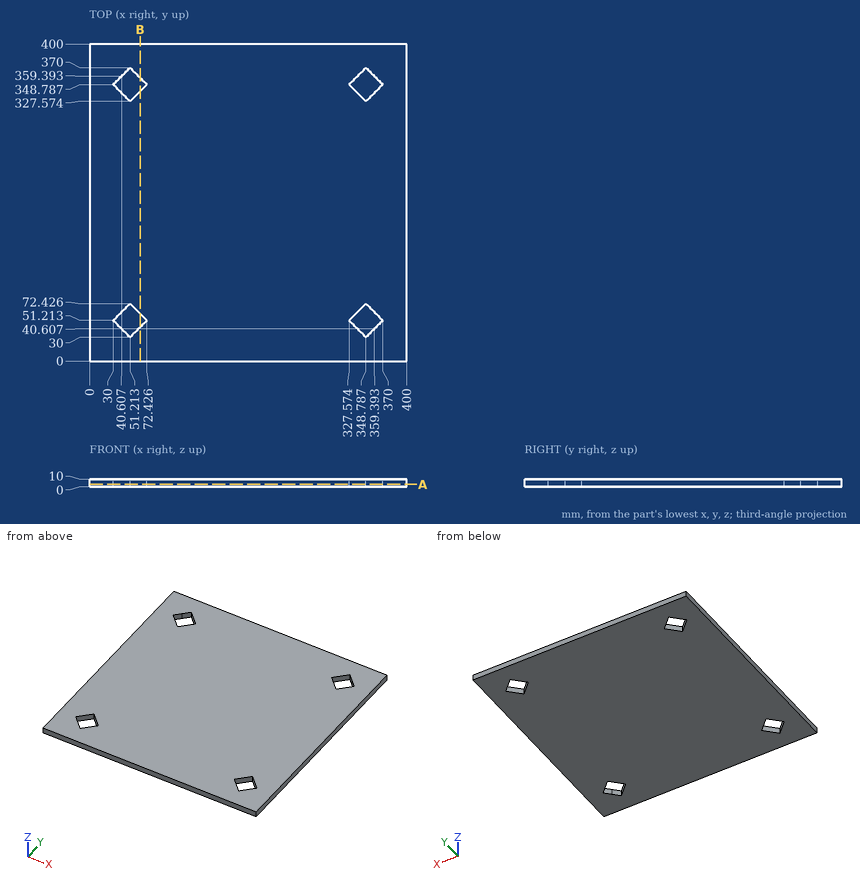
Input: dimensioned drawing with shaded views. Units: mm. Origin: part minimum x, y, z. Give positions to 0.01 mm unless a question says otherwise; leave off trailing zeros. Write each loop counter-clockwise with the first axis right and the second up, starting at its lowest first coordinate (ties: lowest second). Pieces come first, ordered by that corner, then holes. Notation, with made-up numbers: M -8,67 L 21,67 A13 ccw 21,72 Z; hole C 87,21 d7. An arc over 180 degrees is marked long. Return JSON: item names as keys, results as strings. Group by question number.
1) Cut plane B-B, the plane x = 64. Output: boundary loops of the cut face in (y, z).
2) Cut plane A-A, the plane z = 3.25. Output: boundary loops of the cut face in (x, y), plus the area to 3 significant figures.
3) Material intervals for line 1 along Y through (x, z) = (33, 6) (1 decimal); line 2 along Y through (x, z) = (37, 6.5) (1 decimal); line 3 along X through (y, z) = (350.5, 1) (1 decimal), sorted ascending. Write a range as [from, to].
Recorded:
{
 "1": {"outline": "M 0,0 L 42.79,0 L 42.79,10 L 0,10 Z; M 59.64,0 L 340.36,0 L 340.36,10 L 59.64,10 Z; M 357.21,0 L 400,0 L 400,10 L 357.21,10 Z"},
 "2": {"outline": "M 0,0 L 400,0 L 400,400 L 0,400 Z; hole M 30,51.21 L 51.21,30 L 72.43,51.21 L 51.21,72.43 Z; hole M 30,348.79 L 51.21,327.57 L 72.43,348.79 L 51.21,370 Z; hole M 327.57,51.21 L 348.79,30 L 370,51.21 L 348.79,72.43 Z; hole M 327.57,348.79 L 348.79,327.57 L 370,348.79 L 348.79,370 Z", "area": "156,000 mm²"},
 "3": {"line 1": "y = [0, 48.2], [54.2, 345.8], [351.8, 400]", "line 2": "y = [0, 44.2], [58.2, 341.8], [355.8, 400]", "line 3": "x = [0, 31.7], [70.7, 329.3], [368.3, 400]"}
}
